Part model, mm, in its own coordinate system. Give positions to 0.01 mm unless a question says otherwise; leave off trailing zeros. Write each loop counter-clockwise with the first axis right and the second up, starting at its lowest first coordinate (ties: lowest second). Pieces come first, ordered by that corner, then holes.
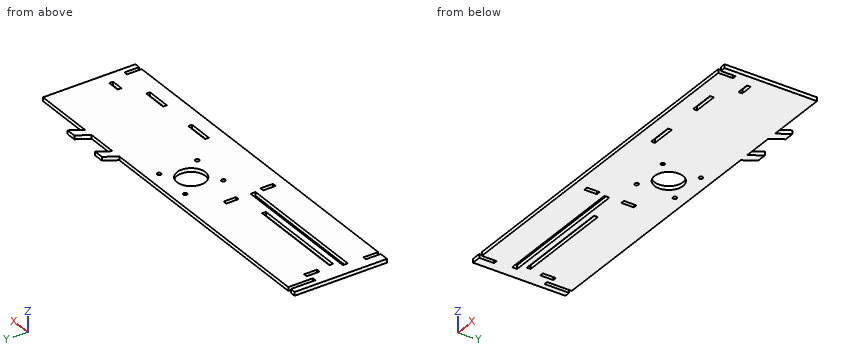
Autodesk Inventor part; units mm, degrees
ref_plane "YZ Plane" through (0, 0, 0) normal (1, 0, 0) x (0, 1, 0)
ref_plane "XZ Plane" through (0, 0, 0) normal (0, 1, 0) x (-1, 0, 0)
ref_plane "XY Plane" through (0, 0, 0) normal (0, 0, 1) x (1, 0, 0)
sketch "Sketch1" plane through (0, 0, 0) normal (0, 0, 1) x (1, 0, 0)
  line L0 (0, 0) -> (300, 0)
  line L1 (300, 0) -> (300, 65)
  line L2 (300, 65) -> (0, 65)
  line L3 (0, 65) -> (0, 0)
  circle A0 centre (144.5, 55.5) radius 1.55
  circle A1 centre (144.5, 24.5) radius 1.55
  circle A2 centre (175.5, 55.5) radius 1.55
  circle A3 centre (175.5, 24.5) radius 1.55
  circle A4 centre (160, 40) radius 11.5
  line L4 (10, 19) -> (120, 19)
  line L5 (120, 19) -> (120, 15)
  line L6 (120, 15) -> (10, 15)
  line L7 (10, 15) -> (10, 19)
  line L8 (0, 65) -> (39.6145, 65)
  line L9 (4.5, 65) -> (7.5, 65)
  line L10 (0, 65) -> (50, 65)
  line L11 (0, 0) -> (0, -10)
  line L12 (0, -10) -> (300, -10)
  line L13 (300, -10) -> (300, 0)
  point P0 (10, 17)
  point P1 (120, 17)
  dimension "d1" = 3.1
  dimension "d2" = 3.1
  dimension "d3" = 3.1
  dimension "d4" = 3.1
  dimension "d5" = 31
  dimension "d7" = 23
  dimension "d8" = 15.5
  dimension "d9" = 15.5
  dimension "d10" = 65
  dimension "d11" = 31
  dimension "d13" = 40
  dimension "d54" = 300
  dimension "d55" = 3
  dimension "d59" = 110
  dimension "d93" = 15
  dimension "d107" = 10
  dimension "d201" = 4
  dimension "d202" = 10
  dimension "d287" = 140
extrude "Extrusion1" add sketch "Sketch1" along normal blind 3
sketch "Sketch7" plane through (0, 0, 3) normal (0, 0, 1) x (1, 0, 0)
  line L0 (300, 65) -> (0, 65)
  circle A0 centre (144.5, 55.5) radius 1.55
  line L1 (118.95, 39.55) -> (122.05, 39.55)
  line L2 (122.05, 39.55) -> (122.05, 29.45)
  line L3 (122.05, 29.45) -> (118.95, 29.45)
  line L4 (118.95, 29.45) -> (118.95, 39.55)
  line L5 (118.95, 39.55) -> (122.05, 29.45) construction
  line L6 (122.05, 39.55) -> (118.95, 29.45) construction
  line L7 (122.1, 9.55) -> (122.1, -0.55)
  line L8 (122.1, -0.55) -> (118.9, -0.55)
  line L9 (118.9, 9.55) -> (122.1, 9.55)
  line L10 (118.9, -0.55) -> (118.9, 9.55)
  line L11 (118.9, 9.55) -> (122.1, -0.55) construction
  line L12 (122.1, 9.55) -> (118.9, -0.55) construction
  line L13 (0, -10) -> (300, -10)
  line L14 (300, -10) -> (300, 65)
  circle A1 centre (144.5, 24.5) radius 1.55
  point P0 (0, 0)
  point P1 (242, 62)
  point P2 (120.5, 34.5)
  point P3 (120.5, 4.5)
  point P4 (118.9, 4.5)
  point P5 (150, -10)
  dimension "d185" = 3.2
  dimension "d271" = 3.1
  dimension "d273" = 30
  dimension "d275" = 24
extrude "Extrusion6" cut sketch "Sketch7" against normal blind 3 contours L1 L2 L3 L4 | L7 L8 L10 L9
sketch "Sketch8" plane through (0, 0, 3) normal (0, 0, 1) x (1, 0, 0)
  line L0 (0, -10) -> (300, -10)
  line L1 (279.95, 18) -> (290, 18)
  line L2 (290, 18) -> (290, 14.95)
  line L3 (290, 14.95) -> (279.95, 14.95)
  line L4 (279.95, 14.95) -> (279.95, 18)
  line L5 (300, -10) -> (300, 65)
  line L6 (7.5, 2) -> (10.5, 2)
  line L7 (10.5, 2) -> (10.5, -10)
  line L8 (10.5, -10) -> (7.5, -10)
  line L9 (7.5, -10) -> (7.5, 2)
  line L10 (7.5, 2) -> (10.5, -10) construction
  line L11 (10.5, 2) -> (7.5, -10) construction
  line L12 (295.5, 2) -> (292.5, 2)
  line L13 (292.5, 2) -> (292.5, -10)
  line L14 (292.5, -10) -> (295.5, -10)
  line L15 (295.5, -10) -> (295.5, 2)
  line L16 (295.5, 2) -> (292.5, -10) construction
  line L17 (292.5, 2) -> (295.5, -10) construction
  line L18 (300, 65) -> (0, 65)
  line L19 (7.5, 45) -> (4.5, 45)
  line L20 (4.5, 45) -> (4.5, 65)
  line L21 (4.5, 65) -> (7.5, 65)
  line L22 (7.5, 65) -> (7.5, 45)
  line L23 (7.5, 45) -> (4.5, 65) construction
  line L24 (4.5, 45) -> (7.5, 65) construction
  point P0 (0, 0)
  point P1 (9, -4)
  point P2 (7.5, -4)
  point P3 (294, -4)
  point P4 (7.5, -10)
  point P5 (10.5, -10)
  point P6 (6, 55)
  dimension "d219" = 28
  dimension "d220" = 3.05
  dimension "d221" = 10.05
  dimension "d222" = 10
  dimension "d223" = 3
  dimension "d247" = 3
  dimension "d248" = 6
  dimension "d249" = 12
  dimension "d296" = 3
  dimension "d297" = 4.5
  dimension "d298" = 20
extrude "Extrusion7" cut sketch "Sketch8" against normal blind 3
sketch "Sketch11" plane through (0, 0, 0) normal (0, 0, -1) x (-1, 0, 0)
  line L0 (-12, 47) -> (-15.05, 47)
  line L1 (-15.05, 47) -> (-15.05, 36.5)
  line L2 (-15.05, 36.5) -> (-12, 36.5)
  line L3 (-12, 36.5) -> (-12, 47)
  line L4 (0, 65) -> (0, -10)
  line L5 (-300, 65) -> (0, 65)
  line L6 (-95.15, 26.5) -> (-15.05, 26.5)
  line L7 (-15.05, 26.5) -> (-15.05, 23.45)
  line L8 (-15.05, 23.45) -> (-95.15, 23.45)
  line L9 (-95.15, 23.45) -> (-95.15, 26.5)
  point P0 (0, 0)
  point P1 (-12, 41.75)
  point P2 (-7.5, 65)
  dimension "d276" = 12
  dimension "d277" = 18
  dimension "d278" = 10.5
  dimension "d279" = 3.05
  dimension "d282" = 10
  dimension "d283" = 80.1
  dimension "d284" = 3.05
extrude "Extrusion9" cut sketch "Sketch11" against normal blind 3
sketch "Sketch12" plane through (0, 0, 3) normal (0, 0, 1) x (1, 0, 0)
  line L0 (194.85, 5.05) -> (214.95, 5.05)
  line L1 (214.95, 5.05) -> (214.95, 2)
  line L2 (214.95, 2) -> (194.85, 2)
  line L3 (194.85, 2) -> (194.85, 5.05)
  line L4 (244.95, 5.05) -> (265, 5.05)
  line L5 (265, 5.05) -> (265, 2)
  line L6 (265, 2) -> (244.95, 2)
  line L7 (244.95, 2) -> (244.95, 5.05)
  point P0 (0, 0)
  point P1 (300, -10)
  dimension "d288" = 3.05
  dimension "d289" = 20.05
  dimension "d290" = 20.1
  dimension "d291" = 30
  dimension "d292" = 35
  dimension "d293" = 12
extrude "Extrusion10" cut sketch "Sketch12" against normal blind 3
sketch "Sketch13" plane through (0, 0, 3) normal (0, 0, 1) x (1, 0, 0)
  line L0 (300, 65) -> (7.5, 65)
  line L1 (209, 65) -> (215, 75)
  line L2 (215, 75) -> (223, 75)
  line L3 (223, 75) -> (217, 65)
  line L4 (242, 65) -> (248, 75)
  line L5 (248, 75) -> (256, 75)
  line L6 (256, 75) -> (250, 65)
  point P0 (0, 0)
  dimension "d299" = 10
  dimension "d300" = 8
  dimension "d301" = 6
  dimension "d302" = 50
  dimension "d303" = 25
  dimension "d304" = 8
extrude "Extrusion11" add sketch "Sketch13" against normal blind 3
properties part number "Sideboard"
1) Saw through at B-B, the plane x = 110.5. Write the cut outline in (y, z), then the cut area to 3 significant figures.
Answers follow:
outline: (-10, 0) - (15, 0) - (15, 3) - (-10, 3) - close; (19, 0) - (65, 0) - (65, 3) - (19, 3) - close
area: 213 mm2
2) Saw through at C-C, the plane z = 1.15. Count the separate pieces of the cut face and the enclosed holes in it, then the cut area to 3 significant figures.
Answers follow:
separate pieces: 1
enclosed holes: 13
area: 21,100 mm2
3) Saw through at A-A, the plane x = 160. Write the cut outline in (y, z), then the cut area to 3 significant figures.
Answers follow:
outline: (-10, 0) - (28.5, 0) - (28.5, 3) - (-10, 3) - close; (51.5, 0) - (65, 0) - (65, 3) - (51.5, 3) - close
area: 156 mm2
4) Wall check: L1, parallel to Y at x = 175.5, z = 1.45; L2, parallel to Y at x = 93, z = 0.35; L3, parallel to X at y = -1.5, z = 1.65. Give the ranges that are in metal, low to high.
Answers follow:
L1: y = -10 to 22.95, 26.05 to 53.95, 57.05 to 65
L2: y = -10 to 15, 19 to 23.45, 26.5 to 65
L3: x = 0 to 7.5, 10.5 to 292.5, 295.5 to 300
5) Pin check, flat tips, straight feed: pin 1 Ø1.9 at (x, y) = (175.5, 55.5) entering from -Z; pin 2 Ø1.5 at (x, z) = (43, 2) entering from +Y; pin 3 Ø1.5 at (x, z) = (6, 1) entering from +Y. Stop position of each tip, or through.
Answers follow:
pin 1: passes through
pin 2: stops at y = 65
pin 3: stops at y = 45
